Geometry check sheet. Reference: the model listing, model coordinates, mm. A direction names the side the tool comes from. Give positions to 0.01 mm unless a question says otherwise; leave off trailing zeros. Loops run counter-clockwise (first coordinate to the right, second up) from the corner with the lowest first, then second, coordinate; pieces in that order, holes last. Notation, with made-up numbers: (31.25, 49.25) -> (43.25, 49.25) arc R28 ccw to (43.25, 75.25) -> close; hole circle Ø8 at (-17, -0.5). An arc over 180 degrees is marked (long way). One line per item, written item: value. Start each with the question number.
(1) Scan lines: line 1 along Z through (x, y) = (0, 1.9); line 2 along Y through (x, z) = (1.75, -1.65); line 3 along X through (y, z) = (3.75, 2.75). Record each from-to range of solid material in increasing order. Write a range as from..to.
(2) Sectioned sample at B-B, the plane y = 3.25. Record the cut outline in (x, z).
(3) Sectioned sample at D-D, the plane z = -2.15. Record the cut outline in (x, y), then the cut area to 3 significant figures.
(4) Gauge pin test, flat ends, axial feed: pin 1 Ø2 at (y, z) = (2.5, -1.5) entering from +X; pin 2 Ø3 at (x, y) = (2, 9.5) entering from -Z; pin 3 Ø2.5 at (x, z) = (-0.5, 0.5) entering from -Y; pin 4 Ø2 at (x, y) = (-2.5, 8.5) entering from +Z. Record the tip position at first contact, or that the pin passes through.
(5) Sectioned sample at C-C, the plane y = 7.25. Record the cut outline in (x, z), then the cut area to 3 significant figures.
(6) Tool access check on faces 1 (the face through (1.438, 2.535, -0.748)), 2 (the face through (-1, 5, 2)), 3 (the face through (0, 2, 3)). Record the directions out of +Z, -Z, +X, -X, +Y, -Y that give a thin tool (end or side, any length) a straight path to the whole face; none if there is none.
(7) Draft check along Z on faces 4 (the face through (0, 8, -2)), 5 (the face through (0, 2, -3)), 6 (the face through (0, 5, 0)). Enter one of: pulls with the +Z half, pulls with the -Z half, needs draft (parallel to the pull), parting line crosses it, or undercut.
(8) Sectioned sample at A-A, the plane x = 0. Record the cut outline in (y, z), then the cut area to 3 significant figures.
Autodesk Inventor part; units mm, degrees
ref_plane "YZ Plane" through (0, 0, 0) normal (1, 0, 0) x (0, 1, 0)
ref_plane "XZ Plane" through (0, 0, 0) normal (0, 1, 0) x (-1, 0, 0)
ref_plane "XY Plane" through (0, 0, 0) normal (0, 0, 1) x (1, 0, 0)
sketch "Sketch1" plane through (0, 0, 0) normal (0, 1, 0) x (-1, 0, 0)
  line L0 (-1.7321, -3) -> (-3.4641, 0)
  line L1 (-3.4641, 0) -> (-1.7321, 3)
  line L2 (-1.7321, 3) -> (1.7321, 3)
  line L3 (1.7321, 3) -> (3.4641, 0)
  line L4 (3.4641, 0) -> (1.7321, -3)
  line L5 (1.7321, -3) -> (-1.7321, -3)
  point P0 (0, 0)
  point P1 (0, 0)
  point P2 (0, 0)
  dimension "d0" = 3
extrude "Extrusion1" add sketch "Sketch1" along normal blind 5
hole "Hole2" at (0, 0, 0) direction (0, 1, 0) diameter 3.242 depth 11.8 tip angle 118
sketch "Sketch3" plane through (0, 5, 0) normal (0, 1, 0) x (1, 0, 0)
  circle A0 centre (0, 0) radius 2
  dimension "d17" = 4
extrude "Extrusion2" add sketch "Sketch3" along normal blind 6
thread "Thread1"
chamfer "Chamfer1" distance 0.7 angle 45 1 edges at (-2, 11, 0)
properties part number "StandoffM4x15B" material "Brass, Soft Yellow"
Calculated:
1. line 1: z = -3..-1.62, 1.62..3
1. line 2: y = 0..5
1. line 3: x = -1.88..1.88
2. outline: (-3.46, 0) -> (-1.73, -3) -> (1.73, -3) -> (3.46, 0) -> (1.73, 3) -> (-1.73, 3) -> close; hole circle Ø3.24 at (0, 0)
3. outline: (-2.22, 0) -> (2.22, 0) -> (2.22, 5) -> (-2.22, 5) -> close
3. area: 22.2 mm2
4. pin 1: stops at x = 3.18
4. pin 2: stops at z = -1.94
4. pin 3: stops at y = 0
4. pin 4: stops at z = 1.32
5. outline: circle Ø4 at (0, 0)
5. area: 12.6 mm2
6. face 1: -Y
6. face 2: +Y
6. face 3: +Z, +X, -X, +Y, -Y
7. face 4: parting line crosses it
7. face 5: pulls with the -Z half
7. face 6: undercut
8. outline: (0, -3) -> (5, -3) -> (5, -2) -> (10.3, -2) -> (11, -1.3) -> (11, 1.3) -> (10.3, 2) -> (5, 2) -> (5, 3) -> (0, 3) -> (0, 1.62) -> (5, 1.62) -> (5, -1.62) -> (0, -1.62) -> close
8. area: 37.3 mm2
